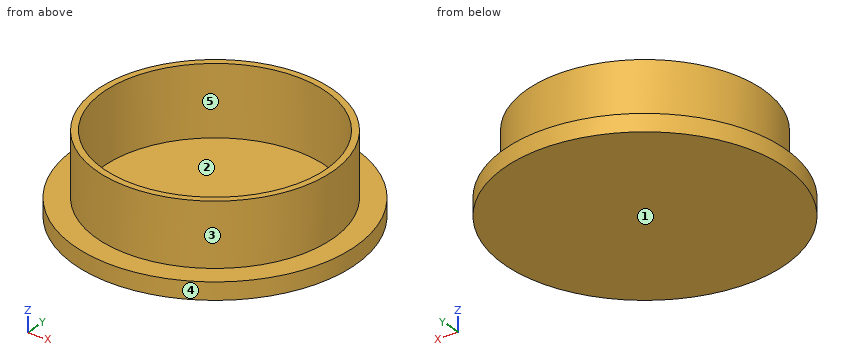
Autodesk Fusion 360 part; units mm, degrees
sketch "Sketch1" plane through (0, 0, 0) normal (0, 0, 1) x (1, 0, 0)
  circle A0 centre (0, 0) radius 30.235
  dimension "d1" = 60.47
extrude "Extrude1" add sketch "Sketch1" along normal blind 3.72
sketch "Sketch2" plane through (0, 0, 3.72) normal (0, 0, 1) x (-1, 0, 0)
  circle A0 centre (0, 0) radius 30.235
  circle A1 centre (0, 0) radius 25.4
  dimension "d4" = 50.8
extrude "Extrude2" add sketch "Sketch2" along normal blind 13.57 contours A1
sketch "Sketch3" plane through (0, 0, 17.29) normal (0, 0, 1) x (-1, 0, 0)
  circle A0 centre (0, 0) radius 25.4
  circle A1 centre (0, 0) radius 24
  dimension "d10" = 48
extrude "Extrude3" cut sketch "Sketch3" against normal blind 15 contours A1
Verification items for the finished model (mm, model axes). Face numbers are marked on the shaded views. A direction names the side the tool comes from. Round coordinates to 2 decimals unless told otherwise and drop trailing zeros. Loops run counter-clockwise (first coordinate to the right, second up) from the corner with the lowest first, then second, coordinate; pieces in that order, holes last. Notation, with made-up numbers: (86, 35) - (129, 35) arc R25 cw to (129, 54) - close; hole circle Ø4 at (85, 71.5). An arc over 180 degrees is marked (long way). Use a Markdown table: item, result. Add a question column.
1. Section check C-C, the plane y = -19. Record the boundary of the cut face in (x, z), plus the area to 3 significant figures.
2. Section check A-A, the plane x = 0. Record the boundary of the cut face in (y, z) (3 decimals).
3. Release check for a two-part mould opening along X. For the marked faces 1, 2 and 3 record: released by +X, released by -X, zero draft, split by the parting line, or undercut.
4. Gauge pin test, flat ends, axial feed: pin 1 (8 mm diameter, centred on x = 6, y = 9.5, fed in from +Z); pin 2 (1 mm diameter, centred on x = -1.5, z = 7.5, fed in from +Y); pin 3 (1.5 mm diameter, centred on y = -22, z = 13.5, fed in from -X). Record the tip position at first contact, or that the pin passes through.
5. Thickness scan on probe 1 along Y at (x, z) = (0, 11.5); probe 2 along Z at (x, y) = (-18, -9). Record the ranges inside material, lowest first. Write a range as [from, to].
6. Access from +Z, -Z, +X, -X, +Y, -Y to the whole of each face (thin tool, end or side, straight path). Record for the marked faces 4 and 5.
7. Section check B-B, the plane z = 14.75. Record the boundary of the cut face in (x, y), plus the area to 3 significant figures.
Checks:
| question | item | result |
|---|---|---|
| 1 | outline | (-23.52, 0) - (23.52, 0) - (23.52, 3.72) - (16.86, 3.72) - (16.86, 17.29) - (14.66, 17.29) - (14.66, 2.29) - (-14.66, 2.29) - (-14.66, 17.29) - (-16.86, 17.29) - (-16.86, 3.72) - (-23.52, 3.72) - close |
| 1 | area | 193 mm^2 |
| 2 | outline | (-30.235, 0) - (30.235, 0) - (30.235, 3.72) - (25.4, 3.72) - (25.4, 17.29) - (24, 17.29) - (24, 2.29) - (-24, 2.29) - (-24, 17.29) - (-25.4, 17.29) - (-25.4, 3.72) - (-30.235, 3.72) - close |
| 3 | face 1 | zero draft |
| 3 | face 2 | undercut |
| 3 | face 3 | split by the parting line |
| 4 | pin 1 | stops at z = 2.29 |
| 4 | pin 2 | stops at y = 25.38 |
| 4 | pin 3 | stops at x = -13.91 |
| 5 | probe 1 | y = [-25.4, -24], [24, 25.4] |
| 5 | probe 2 | z = [0, 2.29] |
| 6 | face 4 | +Z, -Z |
| 6 | face 5 | +Z |
| 7 | outline | circle Ø50.8 at (0, 0); hole circle Ø48 at (0, 0) |
| 7 | area | 217 mm^2 |
